Source: CAD feature listing. Evaluate the final solid. Frame: model axes, mm. A direction names the side the tool comes from. Round coordinates to 2 decimals unless told otherwise and drop trailing zeros. Loops run counter-clockwise (first coordinate to the right, second up) from the corner with the lowest first, then second, coordinate; pieces in that order, holes last. Notation, with made-up numbers: (82.25, -33.75) - (129.25, -33.75) arc R32 ccw to (129.25, -6.75) - close; hole circle Ø3 at (56.25, 46). An arc over 180 degrees is marked (long way). One line per question, with ' | ' between items.
from build123d import *

# Parameters (mm, degrees)
SKETCH1_R           = 1.5
BOSS_EXTRUDE1_DEPTH = 20
CUT_EXTRUDE1_DEPTH  = 2
CUT_EXTRUDE2_START  = 20
CUT_EXTRUDE2_DEPTH  = 2


with BuildPart() as part:
    # Sketch1 → Boss-Extrude1 (new body)
    with BuildSketch(Plane(origin=(0, 0, 0), x_dir=(0, 0, -1), z_dir=(1, 0, 0))):
        with BuildLine():
            Line((-28, 13.216168298), (28, 13.216168298))
            ThreePointArc((28, 13.216168298), (29.414213562, 12.63038186), (30, 11.216168298))
            Line((30, 11.216168298), (30, -11.141664132))
            ThreePointArc((30, -11.141664132), (29.542199202, -12.415093212), (28.378378378, -13.105545442))
            ThreePointArc((28.378378378, -13.105545442), (0, -15.814447135), (-28.378378378, -13.105545442))
            ThreePointArc((-28.378378378, -13.105545442), (-29.542199202, -12.415093212), (-30, -11.141664132))
            Line((-30, -11.141664132), (-30, 11.216168298))
            ThreePointArc((-30, 11.216168298), (-29.414213562, 12.63038186), (-28, 13.216168298))
        make_face()
        with Locations((0, 7.216168298)):
            Circle(SKETCH1_R, mode=Mode.SUBTRACT)
        with Locations((0, -6.783831702)):
            Circle(SKETCH1_R, mode=Mode.SUBTRACT)
        with Locations((-25, 7.216168298)):
            Circle(SKETCH1_R, mode=Mode.SUBTRACT)
        with Locations((-25, -6.783831702)):
            Circle(SKETCH1_R, mode=Mode.SUBTRACT)
        with Locations((25, 7.216168298)):
            Circle(SKETCH1_R, mode=Mode.SUBTRACT)
        with Locations((25, -6.783831702)):
            Circle(SKETCH1_R, mode=Mode.SUBTRACT)
        with BuildLine():
            Line((-20, 6.216168298), (-20, -7.677056726))
            ThreePointArc((-20, -7.677056726), (-19.500582637, -8.999271439), (-18.251748252, -9.661149168))
            ThreePointArc((-18.251748252, -9.661149168), (-12.684282914, -10.258585012), (-7.097902098, -10.640618063))
            ThreePointArc((-7.097902098, -10.640618063), (-5.620834346, -10.091429355), (-5, -8.643015706))
            Line((-5, -8.643015706), (-5, 6.216168298))
            ThreePointArc((-5, 6.216168298), (-5.585786438, 7.63038186), (-7, 8.216168298))
            Line((-7, 8.216168298), (-18, 8.216168298))
            ThreePointArc((-18, 8.216168298), (-19.414213562, 7.63038186), (-20, 6.216168298))
        make_face(mode=Mode.SUBTRACT)
        with BuildLine():
            Line((5, 6.216168298), (5, -8.643015706))
            ThreePointArc((5, -8.643015706), (5.620834346, -10.091429355), (7.097902098, -10.640618063))
            ThreePointArc((7.097902098, -10.640618063), (12.684282914, -10.258585012), (18.251748252, -9.661149168))
            ThreePointArc((18.251748252, -9.661149168), (19.500582637, -8.999271439), (20, -7.677056726))
            Line((20, -7.677056726), (20, 6.216168298))
            ThreePointArc((20, 6.216168298), (19.414213562, 7.63038186), (18, 8.216168298))
            Line((18, 8.216168298), (7, 8.216168298))
            ThreePointArc((7, 8.216168298), (5.585786438, 7.63038186), (5, 6.216168298))
        make_face(mode=Mode.SUBTRACT)
    extrude(amount=BOSS_EXTRUDE1_DEPTH)

    # Sketch2 → Cut-Extrude1 (cut)
    with BuildSketch(Plane(origin=(0, 0, 0), x_dir=(0, 0, -1), z_dir=(1, 0, 0))):
        Polygon((-25, 3.983006791), (-22.2, 5.599587544), (-22.2, 8.832749052), (-25, 10.449329806), (-27.8, 8.832749052), (-27.8, 5.599587544), align=None)
        Polygon((-25, -10.016993209), (-22.2, -8.400412456), (-22.2, -5.167250948), (-25, -3.550670194), (-27.8, -5.167250948), (-27.8, -8.400412456), align=None)
        Polygon((0, 3.983006791), (2.8, 5.599587544), (2.8, 8.832749052), (0, 10.449329806), (-2.8, 8.832749052), (-2.8, 5.599587544), align=None)
        Polygon((0, -10.016993209), (2.8, -8.400412456), (2.8, -5.167250948), (0, -3.550670194), (-2.8, -5.167250948), (-2.8, -8.400412456), align=None)
        Polygon((25, 3.983006791), (27.8, 5.599587544), (27.8, 8.832749052), (25, 10.449329806), (22.2, 8.832749052), (22.2, 5.599587544), align=None)
        Polygon((25, -10.016993209), (27.8, -8.400412456), (27.8, -5.167250948), (25, -3.550670194), (22.2, -5.167250948), (22.2, -8.400412456), align=None)
    extrude(amount=CUT_EXTRUDE1_DEPTH, mode=Mode.SUBTRACT)

    # Sketch2<2> → Cut-Extrude2 (cut)
    with BuildSketch(Plane(origin=(0, 0, 0), x_dir=(0, 0, -1), z_dir=(1, 0, 0)).offset(CUT_EXTRUDE2_START)):
        Polygon((-25, 3.983006791), (-22.2, 5.599587544), (-22.2, 8.832749052), (-25, 10.449329806), (-27.8, 8.832749052), (-27.8, 5.599587544), align=None)
        Polygon((-25, -10.016993209), (-22.2, -8.400412456), (-22.2, -5.167250948), (-25, -3.550670194), (-27.8, -5.167250948), (-27.8, -8.400412456), align=None)
        Polygon((0, 3.983006791), (2.8, 5.599587544), (2.8, 8.832749052), (0, 10.449329806), (-2.8, 8.832749052), (-2.8, 5.599587544), align=None)
        Polygon((0, -10.016993209), (2.8, -8.400412456), (2.8, -5.167250948), (0, -3.550670194), (-2.8, -5.167250948), (-2.8, -8.400412456), align=None)
        Polygon((25, 3.983006791), (27.8, 5.599587544), (27.8, 8.832749052), (25, 10.449329806), (22.2, 8.832749052), (22.2, 5.599587544), align=None)
        Polygon((25, -10.016993209), (27.8, -8.400412456), (27.8, -5.167250948), (25, -3.550670194), (22.2, -5.167250948), (22.2, -8.400412456), align=None)
    extrude(amount=-CUT_EXTRUDE2_DEPTH, mode=Mode.SUBTRACT)


solid = part.part
1. Section query B-B, the plane x = 12.75. Give the number of separate pieces and of enclosed holes in the cut face, plus the area to 3 significant figures.
Worked out:
separate pieces: 1 | enclosed holes: 8 | area: 1,090 mm2
2. Section query C-C, the plane z = 11. Return loops of the section in (x, y).
Worked out:
outline: (0, -15.41) - (20, -15.41) - (20, -10.4) - (0, -10.4) - close; (0, 8.22) - (20, 8.22) - (20, 13.22) - (0, 13.22) - close
3. Access query for faces 4 (the flat face through (2, 5.8, 1.3)), 5 (the flat face through (19.01, 4.78, -1.38)), 6 (the flat face through (10, -1, 5)). Directions: +Z, -Z, +X, -X, +Y, -Y. A direction counts if a zero-diameter tool reaches every point of the face in a straight line with its end or side. Return the directions, or none.
Worked out:
face 4: -X | face 5: +X | face 6: +X, -X
4. Material intervals for probe 1 along Z at (x, y) = (14, -3.25); probe 2 along Y at (x, z) = (6, 25); probe 3 along Z at (x, y) = (5.25, 6.5), sorted ascending.
Worked out:
probe 1: z = -30 to -20, -5 to 5, 20 to 30 | probe 2: y = -13.72 to -8.28, -5.28 to 5.72, 8.72 to 13.22 | probe 3: z = -30 to -26.32, -23.68 to -19.98, -5.02 to -1.32, 1.32 to 5.02, 19.98 to 23.68, 26.32 to 30
5. Contact query for flat-ended pins moving along their axis: P1, Ø12, axis at x = 10.5, z = -14, coming from the -Y side; P2, Ø4, axis at x = 10, z = -22.5, coming from the -Y side; P3, Ø1.7, axis at y = -5.5, z = -1, coming from the +X side. Output: stop coordinate, or through.
Worked out:
P1: stops at y = -15.6 | P2: stops at y = -14.41 | P3: stops at x = 18
6. Mould query, pull axis Y, two halves, no side actions, for faces 1 (the flat face through (10, 0, -30)), 2 (the flat face through (19, -7, 27.8)), 3 (the cylindrical face through (9.86, -12.43, 29.53)). Classes: released by +Y, released by -Y, zero draft, split by the parting line, or undercut.
Worked out:
face 1: zero draft | face 2: undercut | face 3: released by -Y
7. Section query A-A, the plane z = -15.5. Return loops of the section in (x, y), plus the area to 3 significant figures.
Worked out:
outline: (0, -15.01) - (20, -15.01) - (20, -9.98) - (0, -9.98) - close; (0, 8.22) - (20, 8.22) - (20, 13.22) - (0, 13.22) - close | area: 201 mm2
